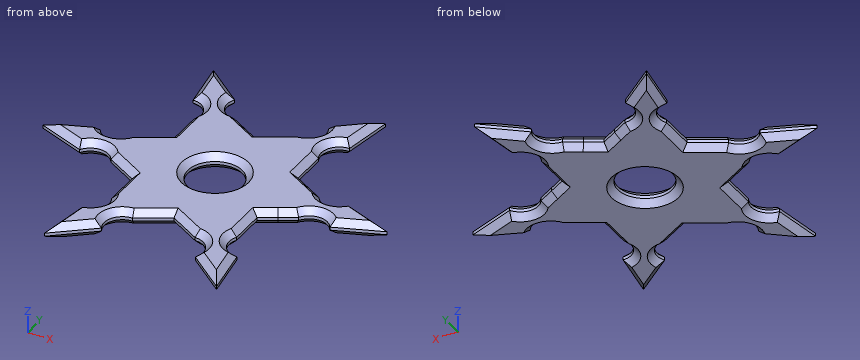
```python
from build123d import *

# Parameters (mm, degrees)
F0_R     = 11
F1_DEPTH = 6.35
F2_SIZE  = 2.54


with BuildPart() as f1:
    # F0 (on Top) → F1 (new body)
    with BuildSketch(Plane.XY):
        Polygon((-41.7423269987, 30.386245353), (-16.3423269987, 45.0509421904), (-22.6923274444, 48.717116657), (-29.0423278901, 52.3832911237), (-41.7423269987, 45.0509425335), (-41.7423269987, 37.7185939432), align=None)
        Polygon((9.0576730013, 1.0568516781), (9.0576730013, 30.386245353), (-16.3423269987, 45.0509421904), (-41.7423269987, 30.386245353), (-41.7423269987, 1.0568516781), (-16.3423269987, -13.6078451593), align=None)
        with Locations((-16.3423269987, 15.7215485155)):
            Circle(F0_R, mode=Mode.SUBTRACT)
        Polygon((-41.7423269987, 1.0568516781), (-41.7423269987, 30.386245353), (-48.092324038, 26.720072853), (-54.4423210773, 23.053900353), (-54.4423210773, 8.3891966781), (-48.092324038, 4.7230241781), align=None)
        Polygon((-22.692324038, -17.2740176593), (-16.3423269987, -13.6078451593), (-41.7423269987, 1.0568516781), (-41.7423269987, -6.2754933219), (-41.7423269987, -13.6078383219), (-29.0423210773, -20.9401901593), align=None)
        Polygon((9.0576730013, -6.2754933219), (9.0576730013, 1.0568516781), (-16.3423269987, -13.6078451593), (-9.9923299594, -17.2740176593), (-3.6423329201, -20.9401901593), (9.0576730013, -13.6078383219), align=None)
        Polygon((15.4076717053, 26.7200718918), (9.0576730013, 30.386245353), (9.0576730013, 1.0568516781), (15.4076710394, 4.7230247548), (21.7576690776, 8.3891978315), (21.7576704094, 23.0538984307), align=None)
        Polygon((-16.3423269987, 45.0509421904), (9.0576730013, 30.386245353), (9.0576730013, 37.7185939432), (9.0576730013, 45.0509425335), (-3.6423261074, 52.3832911237), (-9.992326553, 48.717116657), align=None)
        Polygon((-35.3923274444, 63.381813666), (-51.2673278158, 76.2134228412), (-41.7423271473, 59.7156392851), align=None)
        Polygon((-41.7423271473, 59.7156392851), (-51.2673278158, 76.2134228412), (-48.0923268502, 56.0494649042), align=None)
        with BuildLine():
            Line((-41.7423269987, 45.0509425335), (-29.0423278901, 52.3832911237))
            ThreePointArc((-29.0423278901, 52.3832911237), (-35.3923274939, 56.0494655046), (-35.3923274444, 63.381813666))
            Line((-35.3923274444, 63.381813666), (-41.7423271473, 59.7156392851))
            Line((-41.7423271473, 59.7156392851), (-48.0923268502, 56.0494649042))
            ThreePointArc((-48.0923268502, 56.0494649042), (-41.7423271473, 52.3832906948), (-41.7423269987, 45.0509425335))
        make_face()
        Polygon((-67.1423210773, 23.053900353), (-86.1923210773, 15.7215485155), (-67.1423210773, 15.7215485155), align=None)
        Polygon((-67.1423210773, 15.7215485155), (-86.1923210773, 15.7215485155), (-67.1423210773, 8.3891966781), align=None)
        with BuildLine():
            Line((-54.4423210773, 8.3891966781), (-54.4423210773, 23.053900353))
            ThreePointArc((-54.4423210773, 23.053900353), (-60.7923210773, 19.3877261436), (-67.1423210773, 23.053900353))
            Line((-67.1423210773, 23.053900353), (-67.1423210773, 15.7215485155))
            Line((-67.1423210773, 15.7215485155), (-67.1423210773, 8.3891966781))
            ThreePointArc((-67.1423210773, 8.3891966781), (-60.7923210773, 12.0553708875), (-54.4423210773, 8.3891966781))
        make_face()
        with BuildLine():
            ThreePointArc((-35.3923210773, -31.9387127874), (-35.3923181166, -24.606366078), (-29.0423210773, -20.9401901593))
            Line((-29.0423210773, -20.9401901593), (-41.7423269987, -13.6078383219))
            ThreePointArc((-41.7423269987, -13.6078383219), (-41.7423284791, -20.9401858859), (-48.0923269987, -24.6063609499))
            Line((-48.0923269987, -24.6063609499), (-41.742324038, -28.2725368686))
            Line((-41.742324038, -28.2725368686), (-35.3923210773, -31.9387127874))
        make_face()
        Polygon((-48.0923269987, -24.6063609499), (-51.267324038, -44.7703208107), (-41.742324038, -28.2725368686), align=None)
        Polygon((-51.267324038, -44.7703208107), (-35.3923210773, -31.9387127874), (-41.742324038, -28.2725368686), align=None)
        Polygon((18.5826774423, -44.7703233748), (15.4076848441, -24.6063609499), (9.0576774423, -28.2725394327), align=None)
        Polygon((2.7076700406, -31.9387179154), (18.5826774423, -44.7703233748), (9.0576774423, -28.2725394327), align=None)
        with BuildLine():
            ThreePointArc((15.4076848441, -24.6063609499), (9.0576744816, -20.9401927233), (9.0576730013, -13.6078383219))
            Line((9.0576730013, -13.6078383219), (-3.6423329201, -20.9401901593))
            ThreePointArc((-3.6423329201, -20.9401901593), (2.7076700406, -24.606366078), (2.7076700406, -31.9387179154))
            Line((2.7076700406, -31.9387179154), (9.0576774423, -28.2725394327))
            Line((9.0576774423, -28.2725394327), (15.4076848441, -24.6063609499))
        make_face()
        Polygon((34.457666414, 8.3891966781), (53.5076670799, 15.7215485155), (34.4576670799, 15.7215485155), align=None)
        with BuildLine():
            ThreePointArc((34.4576677458, 23.053900353), (28.1076696325, 19.3877274892), (21.7576704094, 23.0538984307))
            Line((21.7576704094, 23.0538984307), (21.7576690776, 8.3891978315))
            ThreePointArc((21.7576690776, 8.3891978315), (28.1076680788, 12.0553691574), (34.457666414, 8.3891966781))
            Line((34.457666414, 8.3891966781), (34.4576670799, 15.7215485155))
            Line((34.4576670799, 15.7215485155), (34.4576677458, 23.053900353))
        make_face()
        Polygon((34.4576670799, 15.7215485155), (53.5076670799, 15.7215485155), (34.4576677458, 23.053900353), align=None)
        with BuildLine():
            Line((-3.6423261074, 52.3832911237), (9.0576730013, 45.0509425335))
            ThreePointArc((9.0576730013, 45.0509425335), (9.0576733974, 52.3832904375), (15.4076728527, 56.0494645611))
            Line((15.4076728527, 56.0494645611), (9.0576723328, 59.7156394138))
            Line((9.0576723328, 59.7156394138), (2.7076718128, 63.3818142664))
            ThreePointArc((2.7076718128, 63.3818142664), (2.7076727042, 56.0494663623), (-3.6423261074, 52.3832911237))
        make_face()
        Polygon((9.0576723328, 59.7156394138), (18.5826730013, 76.2134229699), (2.7076718128, 63.3818142664), align=None)
        Polygon((9.0576723328, 59.7156394138), (15.4076728527, 56.0494645611), (18.5826730013, 76.2134229699), align=None)
    extrude(amount=F1_DEPTH)

    # F2
    f2_edges = [f1.edges().sort_by_distance(p)[0] for p in [
        (-41.742327, 37.718594, 6.35),
        (-48.092324, 26.720073, 6.35),
        (-60.792321, 19.387726, 6.35),
        (-76.667321, 19.387724, 6.35),
        (-76.667321, 12.055373, 6.35),
        (-60.792321, 12.055371, 6.35),
        (-48.092324, 4.723024, 6.35),
        (-41.742327, -6.275493, 6.35),
        (-41.742328, -20.940186, 6.35),
        (-49.679826, -34.688341, 6.35),
        (-43.329823, -38.354517, 6.35),
        (-35.392318, -24.606366, 6.35),
        (-22.692324, -17.274018, 6.35),
        (-9.99233, -17.274018, 6.35),
        (2.70767, -24.606366, 6.35),
        (10.645174, -38.354521, 6.35),
        (16.995181, -34.688342, 6.35),
        (9.057674, -20.940193, 6.35),
        (9.057673, -6.275493, 6.35),
        (15.407671, 4.723025, 6.35),
        (28.107668, 12.055369, 6.35),
        (43.982667, 12.055373, 6.35),
        (43.982667, 19.387724, 6.35),
        (28.10767, 19.387727, 6.35),
        (15.407672, 26.720072, 6.35),
        (9.057673, 37.718594, 6.35),
        (9.057673, 52.38329, 6.35),
        (16.995173, 66.131444, 6.35),
        (10.645172, 69.797619, 6.35),
        (2.707673, 56.049466, 6.35),
        (-9.992327, 48.717117, 6.35),
        (-22.692327, 48.717117, 6.35),
        (-35.392327, 56.049466, 6.35),
        (-43.329828, 69.797618, 6.35),
        (-49.679827, 66.131444, 6.35),
        (-41.742327, 52.383291, 6.35),
        (-27.342327, 15.721549, 6.35),
        (-41.742327, 37.718594, 0),
        (-48.092324, 26.720073, 0),
        (-60.792321, 19.387726, 0),
        (-76.667321, 19.387724, 0),
        (-76.667321, 12.055373, 0),
        (-60.792321, 12.055371, 0),
        (-48.092324, 4.723024, 0),
        (-41.742327, -6.275493, 0),
        (-41.742328, -20.940186, 0),
        (-49.679826, -34.688341, 0),
        (-43.329823, -38.354517, 0),
        (-35.392318, -24.606366, 0),
        (-22.692324, -17.274018, 0),
        (-9.99233, -17.274018, 0),
        (2.70767, -24.606366, 0),
        (10.645174, -38.354521, 0),
        (16.995181, -34.688342, 0),
        (9.057674, -20.940193, 0),
        (9.057673, -6.275493, 0),
        (15.407671, 4.723025, 0),
        (28.107668, 12.055369, 0),
        (43.982667, 12.055373, 0),
        (43.982667, 19.387724, 0),
        (28.10767, 19.387727, 0),
        (15.407672, 26.720072, 0),
        (9.057673, 37.718594, 0),
        (9.057673, 52.38329, 0),
        (16.995173, 66.131444, 0),
        (10.645172, 69.797619, 0),
        (2.707673, 56.049466, 0),
        (-9.992327, 48.717117, 0),
        (-22.692327, 48.717117, 0),
        (-35.392327, 56.049466, 0),
        (-43.329828, 69.797618, 0),
        (-49.679827, 66.131444, 0),
        (-41.742327, 52.383291, 0),
        (-27.342327, 15.721549, 0),
    ]]
    chamfer(f2_edges, length=F2_SIZE)


solid = f1.part
```
Input: part model. Units: mm. Frame: model coordinates. Give positions to 0.01 mm unless a question says otherwise; leave off trailing zeros. Order: outer loops, then holes, each group sorted by start corner. A loop starts at its lowest first (then second) coordinate and runs counter-clockwise, first axis right, second up. Notation, with made-up numbers: M 88.5,34 L 141.5,34 A23 ccw 141.5,45 Z; hole C 61,-10.75 d3. An arc over 180 degrees is marked long. Return JSON: item names as keys, results as strings.
Item 1: Cut plane C-C (x = -70.5). Return loops of the section in (y, z), then the cut area to 3 significant figures.
Solutions:
{"outline": "M 9.68,2.54 L 12.4,0 L 19.04,0 L 21.76,2.54 L 21.76,3.81 L 19.04,6.35 L 12.4,6.35 L 9.68,3.81 Z", "area": "62.9 mm^2"}
Item 2: Ray query, probe 1 along Y at (x, z) = (-47, 4.75); probe 2 along X at (y, z) = (-39, 4); probe 3 along Y at (x, z) = (-56, 3.5). Return the intervals inside material, ascending.
Solutions:
{"probe 1": "-40.11 to -25.47, 5.18 to 26.27, 56.92 to 71.56", "probe 2": "-50.17 to -44.43, 11.75 to 17.48", "probe 3": "10.27 to 21.17"}
Item 3: First-contact query: P1, Ø1.4, axis at y = -8.5, z = 3, coming from the -X side; P2, Ø1.5, axis at x = -70, z = 3, coming from the -Y side; P3, Ø3, axis at y = -16.5, z = 1, coming from the +X side. Flat tips, straight axial feed; report the tip coordinate or a pass-through.
Solutions:
{"P1": "x = -41.74", "P2": "y = 9.2", "P3": "x = 8.09"}
Item 4: Cut plane B-B (y = 66). Return loops of the section in (x, z).
Solutions:
{"outline": "M -49.66,2.54 L -47.09,0 L -42.67,0 L -38.63,2.54 L -38.63,3.81 L -42.67,6.35 L -47.09,6.35 L -49.66,3.81 Z; M 5.95,2.54 L 9.99,0 L 14.4,0 L 16.97,2.54 L 16.97,3.81 L 14.4,6.35 L 9.99,6.35 L 5.95,3.81 Z"}
Item 5: Cut plane A-A (y = -1). Return loops of the section in (x, z), then the cut area to 3 significant figures.
Solutions:
{"outline": "M -41.74,2.54 L -39.2,0 L 6.52,0 L 9.06,2.54 L 9.06,3.81 L 6.52,6.35 L -39.2,6.35 L -41.74,3.81 Z", "area": "310 mm^2"}
